Build history of the part. All positions in model axes, mm. A direction names the side the tool comes from. Coordinates: 2 decimals unless noted, no trailing zeros. Write each loop counter-clockwise with the first axis right and the second up, starting at its lowest first coordinate (ties: lowest second). Pieces come first, ordered by that corner, then holes. Notation, with made-up numbers: (9, 76.5) -> (35, 76.5) arc R9 ccw to (35, 87.5) -> close; hole circle Ø3 at (51, -6). An arc over 180 degrees is marked (long way). Write each question's results on one line, items separated by ' | '. Start each with the question number.
Q1. Two-plate mould, pull along Y, no slides. Class faces 3 (the face through (14, -313, 25.4)), 4 (the face through (25.48, -331.45, 1.61)), 5 (the face through (25, -635, 23)): released by +Y, released by -Y, zero draft, split by the parting line, or undercut.
Q2. Drill centre lines: line 1 (Z direction, x = 45, y = -67.5) (3 decimals); line 2 (Y direction, x = 25.4, z = 24.7); line 3 (X direction, y = -578.5, z = 7) (3 decimals). Where is each one in solid material? Low to high.
Q3. Saw through at A-A on z = 8.25. Give the cut face in (x, y) (3 decimals), and give its area (3 significant figures).
Q4. Saw through at D-D on x = 20. Count the separate pieces of the cut face and the enclosed holes in it, and give its area (3 significant figures).
Q5. Saw through at B-B on y = -317.5. Give the cut face in (x, z) (1 decimal).
Q6. Tool access for faces 1 (the face through (14, -313, 0)), 2 (the face through (10, -313, 22.225)): list every direction of +Z, -Z, +X, -X, +Y, -Y with a clear straight run to the whole face (end or side of a thin tool).
Q7. Drop a flat-ended pin along its axis: pin 1 Ø4 at (x, z) = (13, 19.5) entering from -Y. Give the stop position or say it passes through.
Q8. Saw through at C-C on y = -439.5. Give the cut face in (x, z) (3 decimals), and give its area (3 significant figures).
from build123d import *

# Parameters (mm, degrees)
F0_W     = 50.8
F0_H     = 25.4
F0_W_2   = 44.45
F0_H_2   = 19.05
F1_DEPTH = 635
F2_R     = 14.2875
F3_DEPTH = 25.401


with BuildPart() as f1:
    # F0 (on Front) → F1 (new body)
    with BuildSketch(Plane.XZ):
        with Locations((25.4, 12.7)):
            Rectangle(F0_W, F0_H)
        with Locations((25.4, 12.7)):
            Rectangle(F0_W_2, F0_H_2, mode=Mode.SUBTRACT)
    extrude(amount=F1_DEPTH)

    # F2 (on face) → F3 (cut, through all)
    with BuildSketch(Plane.XY.offset(25.4)):
        with Locations((25.4, -38.11804)):
            Circle(F2_R)
        with Locations((28.575, -317.5)):
            Circle(F2_R)
        with Locations((25.4, -596.88196)):
            Circle(F2_R)
    extrude(amount=-F3_DEPTH, mode=Mode.SUBTRACT)


solid = f1.part
Returned:
1) face 3: zero draft | face 4: undercut | face 5: released by -Y
2) line 1: z = 0 to 3.175, 22.225 to 25.4 | line 2: y = -635 to -611.17, -582.59 to -331.43, -303.57 to -52.41, -23.83 to 0 | line 3: x = 0 to 3.175, 47.625 to 50.8
3) outline: (0, -635) -> (3.175, -635) -> (3.175, 0) -> (0, 0) -> close; (47.625, -635) -> (50.8, -635) -> (50.8, 0) -> (47.625, 0) -> close | area: 4,030 mm2
4) separate pieces: 8 | enclosed holes: 0 | area: 3,550 mm2
5) outline: (0, 0) -> (14.3, 0) -> (14.3, 3.2) -> (3.2, 3.2) -> (3.2, 22.2) -> (14.3, 22.2) -> (14.3, 25.4) -> (0, 25.4) -> close; (42.9, 0) -> (50.8, 0) -> (50.8, 25.4) -> (42.9, 25.4) -> (42.9, 22.2) -> (47.6, 22.2) -> (47.6, 3.2) -> (42.9, 3.2) -> close
6) face 1: -Z, +X, -X, +Y, -Y | face 2: +Y, -Y
7) pin 1: passes through
8) outline: (0, 0) -> (50.8, 0) -> (50.8, 25.4) -> (0, 25.4) -> close; hole (3.175, 3.175) -> (47.625, 3.175) -> (47.625, 22.225) -> (3.175, 22.225) -> close | area: 444 mm2
